Can you work these out from the model? Positions are in its coordinate system, mm. A direction names the side the tool comes from. Round coordinates to 2 decimals unless told otherwise and drop trailing zeros. Order: outer loops, then holes, each group sorted by start corner. A loop starts at its lowest first (then second) coordinate and runs counter-clockwise, first axis right, second up. Notation, with made-up numbers: M 32,6.5 L 39,6.5 A28 cw 39,25.5 Z; hole C 29,38.5 d8. An arc over 180 degrees is marked long. One line per question, with ' | ' between items.
Autodesk Inventor part; units mm, degrees
ref_plane "YZ Plane" through (0, 0, 0) normal (1, 0, 0) x (0, 1, 0)
ref_plane "XZ Plane" through (0, 0, 0) normal (0, 1, 0) x (-1, 0, 0)
ref_plane "XY Plane" through (0, 0, 0) normal (0, 0, 1) x (1, 0, 0)
sketch "Sketch1" plane through (0, 0, 0) normal (0, 1, 0) x (-1, 0, 0)
  line L0 (18.5932, 129.0225) -> (-51.4068, 129.0225)
  line L1 (-51.4068, 129.0225) -> (-51.4068, -40.9775)
  line L2 (-51.4068, -40.9775) -> (18.5932, -40.9775)
  line L3 (18.5932, -40.9775) -> (18.5932, 129.0225)
  line L4 (-3.9068, 129.0225) -> (-28.9068, 129.0225)
  line L5 (-28.9068, 129.0225) -> (-28.9068, 134.0225)
  line L6 (-28.9068, 134.0225) -> (-3.9068, 134.0225)
  line L7 (-3.9068, 134.0225) -> (-3.9068, 129.0225)
  line L8 (-3.9068, -40.9775) -> (-28.9068, -40.9775)
  line L9 (-28.9068, -40.9775) -> (-28.9068, -45.9775)
  line L10 (-28.9068, -45.9775) -> (-3.9068, -45.9775)
  line L11 (-3.9068, -45.9775) -> (-3.9068, -40.9775)
  point P0 (0, 0)
  dimension "d0" = 70
  dimension "d1" = 170
  dimension "d2" = 25
  dimension "d3" = 5
  dimension "d4" = 22.5
  dimension "d5" = 25
  dimension "d6" = 5
extrude "Extrusion1" add sketch "Sketch1" along normal blind 5
equation "\"d4\" = -0.5 * d2 + 0.5 * d0"
properties part number "piso medio"
(1) Please list where this line runs through material, in increasing order: probe 1 along Z at (x, y) = (-2, 2.25). Write a range as [from, to].
Final values:
probe 1: [-40.98, 129.02]
(2) On a 3-axis mill with a long thin cutter (end or side, diameter ignored), from which of +Z, -Z, +X, -X, +Y, -Y can I reach the whole of each face in a straight line? I mean faces 1 (the flat face through (-8, 2, 129.023)), 2 (the flat face through (-7, 2, -40.978)), 3 (the flat face through (28.907, 2, 131)). Say none if no direction works.
Final values:
face 1: +Z, -X, +Y, -Y | face 2: -Z, -X, +Y, -Y | face 3: +Z, +X, +Y, -Y
(3) Will these pins go through, and if not, where does the flat tip stop? pin 1 Ø1.5 at (y, z) = (3.5, 131.5) entering from +X; pin 2 Ø2.5 at (x, y) = (-9, 3) entering from +Z; pin 3 Ø1.5 at (x, y) = (41, 2) entering from -Z.
Final values:
pin 1: x = 28.91 | pin 2: z = 129.02 | pin 3: z = -40.98
(4) If we section it at B-B on x = -11.5: Please give me the cut outline in (y, z), plus the area to 3 significant figures.
Final values:
outline: M 0,-40.98 L 5,-40.98 L 5,129.02 L 0,129.02 Z | area: 850 mm^2
(5) If we section it at A-A on y = 2.4: Please give me the cut outline in (x, z), plus the area to 4 significant figures.
Final values:
outline: M -18.59,-40.98 L 3.91,-40.98 L 3.91,-45.98 L 28.91,-45.98 L 28.91,-40.98 L 51.41,-40.98 L 51.41,129.02 L 28.91,129.02 L 28.91,134.02 L 3.91,134.02 L 3.91,129.02 L -18.59,129.02 Z | area: 12,150 mm^2
